Check sheet for the modelled part. Datum: model origin and axes. Units: mm. Face numbers are marked on the shaded views. Give positions to 0.01 mm unless a question says otherwise; leave off trailing zeros. Order: outer loops, then holes, each group sorted by start corner. A loop starts at its lowest first (then second) coordinate and runs counter-clockwise, first axis right, second up. Notation, with made-up numbers: M 17,77 L 29,77 A36 ccw 29,115 Z; hole C -10,-8.75 d4. An arc over 180 degrees is marked long. Return JSON: item names as keys, results as strings. Group by question number.
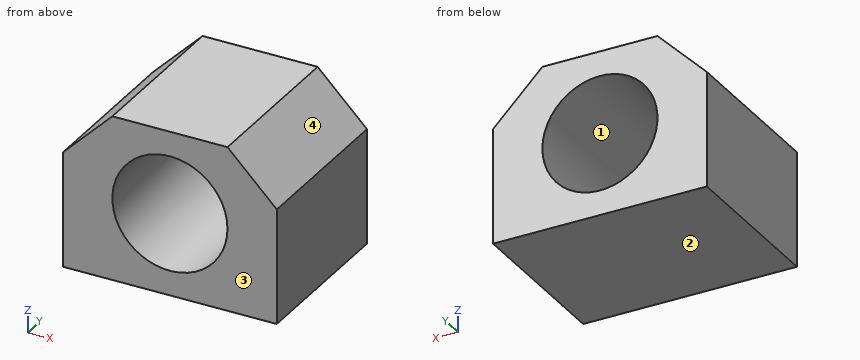
from build123d import *

# Parameters (mm, degrees)
F0_R     = 14
F1_DEPTH = 40


with BuildPart() as f1:
    # F0 (on Front) → F1 (new body)
    with BuildSketch(Plane.XZ):
        Polygon((13.999691, 20), (-14, 20), (-26, 7.999382), (-26, -20), (26, -20), (26, 7.999691), align=None)
        Circle(F0_R, mode=Mode.SUBTRACT)
    extrude(amount=-F1_DEPTH)


solid = f1.part
1) Release check for a two-part mould opening along Z. For the marked faces 1, 2, 3 and 4 record: released by +Z, released by -Z, zero draft, split by the parting line, or undercut.
2) Sectioned sample at B-B on z = 0. Record the boundary of the cut face in (x, y), then the cut area to 3 significant figures.
3) Sectioned sample at C-C on y = 16.5. Record the boundary of the cut face in (x, z), then the cut area to 3 significant figures.
4) Sectioned sample at A-A on x = 0. Record the boundary of the cut face in (y, z).
5) Depth check by flat-ended pin: P1, Ø3, axis at y = 34.5, z = 15.5, coming from the +X side. Enter the tip coordinate at first touch or a pass-through.
6) Material ranges on line 1 along Z through (x, y) = (0, 16); line 2 along X through (y, z) = (14, 1); line 3 along X through (y, z) = (6.5, 13), recorded low to high.
7) Sectioned sample at D-D on x = 20. Record the boundary of the cut face in (y, z), then the cut area to 3 significant figures.
Reply:
{
 "1": {"face 1": "undercut", "face 2": "released by -Z", "face 3": "zero draft", "face 4": "released by +Z"},
 "2": {"outline": "M -26,0 L -14,0 L -14,40 L -26,40 Z; M 14,0 L 26,0 L 26,40 L 14,40 Z", "area": "960 mm^2"},
 "3": {"outline": "M -26,-20 L 26,-20 L 26,8 L 14,20 L -14,20 L -26,8 Z; hole C 0,0 d28", "area": "1,320 mm^2"},
 "4": {"outline": "M 0,-20 L 40,-20 L 40,-14 L 0,-14 Z; M 0,14 L 40,14 L 40,20 L 0,20 Z"},
 "5": {"P1": "x = 20"},
 "6": {"line 1": "-20 to -14, 14 to 20", "line 2": "-26 to -13.96, 13.96 to 26", "line 3": "-21 to -5.2, 5.2 to 21"},
 "7": {"outline": "M 0,-20 L 40,-20 L 40,14 L 0,14 Z", "area": "1,360 mm^2"}
}
